```python
from build123d import *

# Parameters (mm, degrees)
CROQUIS2_W                   = 20
CROQUIS2_H                   = 20
SALIENTE_EXTRUIR1_DEPTH      = 50
CROQUIS3_W                   = 20
CROQUIS3_H                   = 20
SALIENTE_EXTRUIR2_DEPTH      = 59
SALIENTE_EXTRUIR4_DEPTH      = 60
SALIENTE_EXTRUIR4_DEPTH_BACK = 20
CROQUIS7_W                   = 30
CROQUIS7_H                   = 10
CROQUIS14_R                  = 12.5
CORTAR_EXTRUIR4_DEPTH        = 5
CROQUIS16_R                  = 2.25
CORTAR_EXTRUIR5_DEPTH        = 10
CROQUIS19_R                  = 1.65
CORTAR_EXTRUIR6_DEPTH        = 10


with BuildPart() as part:
    # Croquis2 → Saliente-Extruir1 (new body)
    with BuildSketch(Plane.XY):
        Rectangle(CROQUIS2_W, CROQUIS2_H)
    extrude(amount=SALIENTE_EXTRUIR1_DEPTH)

    # Croquis3 → Saliente-Extruir2 (add)
    with BuildSketch(Plane(origin=(0, 10, 0), x_dir=(1, 0, 0), z_dir=(0, 1, 0))):
        with Locations((0, -40)):
            Rectangle(CROQUIS3_W, CROQUIS3_H)
    extrude(amount=SALIENTE_EXTRUIR2_DEPTH)

    # Croquis7 → Saliente-Extruir4 (add, two sides: drawn at the far end of the back side and taken through both)
    with BuildSketch(Plane(origin=(0, 0, 30), x_dir=(-1, 0, 0), z_dir=(0, 0, -1)).offset(-SALIENTE_EXTRUIR4_DEPTH_BACK)):
        with Locations((0, 64)):
            Rectangle(CROQUIS7_W, CROQUIS7_H)
    extrude(amount=SALIENTE_EXTRUIR4_DEPTH + SALIENTE_EXTRUIR4_DEPTH_BACK)

    # Croquis14 → Cortar-Extruir4 (cut)
    with BuildSketch(Plane(origin=(0, 69, 0), x_dir=(1, 0, 0), z_dir=(0, 1, 0))):
        with Locations(Location((0, 0, 0), (0, 0, 270))):
            Circle(CROQUIS14_R)
    extrude(amount=-CORTAR_EXTRUIR4_DEPTH, mode=Mode.SUBTRACT)

    # Croquis16 → Cortar-Extruir5 (cut)
    with BuildSketch(Plane(origin=(0, 64, 0), x_dir=(1, 0, 0), z_dir=(0, 1, 0))):
        with Locations(Location((0, 0, 0), (0, 0, 270))):
            Circle(CROQUIS16_R)
    extrude(amount=-CORTAR_EXTRUIR5_DEPTH, mode=Mode.SUBTRACT)

    # Croquis19 → Cortar-Extruir6 (cut)
    with BuildSketch(Plane(origin=(0, 64, 0), x_dir=(1, 0, 0), z_dir=(0, 1, 0))):
        with Locations(Location((8.5, 0, 0), (0, 0, 270))):
            Circle(CROQUIS19_R)
        with Locations(Location((-8.5, 0, 0), (0, 0, 90))):
            Circle(CROQUIS19_R)
    extrude(amount=-CORTAR_EXTRUIR6_DEPTH, mode=Mode.SUBTRACT)


solid = part.part
```
Geometry check sheet. Reference: the model listing, model coordinates, mm. A direction names the side the tool comes from. Coordinates: 2 decimals unless noted, no trailing zeros. Order: outer loops, then holes, each group sorted by start corner. A loop starts at its lowest first (then second) coordinate and runs counter-clockwise, first axis right, second up. Notation, with made-up numbers: (56.5, -0.5) - (77.5, -0.5) arc R8 cw to (77.5, 13.5) - close; hole circle Ø10 at (66.5, -31.75). An arc over 180 degrees is marked (long way). Answer as a JSON object with one key per item and string values. Group by question number.
Item 1: Sectioned sample at C-C, the plane y = -2. Record the cut outline in (x, z), and give its area (3 significant figures).
Item 2: Sectioned sample at B-B, the plane x = 8.5. Record the cut outline in (y, z).
Item 3: Tool access check on faces 1 (the face through (-10, 16, 31)), 2 (the face through (0, 0, 0)), 3 (the face through (3.755, 66.535, 11.923)), 4 (the face through (0, 10, 15)), 5 (the face through (10, 16, 31)). Record the directions out of +Z, -Z, +X, -X, +Y, -Y that give a thin tool (end or side, any length) a straight path to the whole face; none if there is none.
Item 4: Depth check by flat-ended pin: pin 1 Ø2 at (x, y) = (-5, 22.5) entering from -Z; pin 2 Ø10 at (x, y) = (-3.5, 3.5) entering from -Z; pin 3 Ø2 at (x, z) = (8.5, 0) entering from +Y; pin 4 Ø4 at (x, y) = (6, 58) entering from -Z. Enter the tip coordinate at first touch or a pass-through.
Item 5: Sectioned sample at D-D, the plane z = 38. Record the cut outline in (x, y), and give its area (3 significant figures).
Item 6: Sectioned sample at A-A, the plane z = 18. Record the cut outline in (x, y), and give its area (3 significant figures).
Item 7: Draft check along Y on faces 6 (the face through (4, 59, 2)), 7 (the face through (0, 34, 30)), 8 (the face through (15, 64, 11)), 9 (the face through (0, 64, 3)). Enter one of: +Y half, -Y half, draft (parallel to the pull), parting line (faces both ways), or undercut.
Item 8: Scan lines: probe 1 along X at (y, z) = (62.25, 0); probe 2 along Y at (x, z) = (9, 19); probe 3 along Z at (x, y) = (3.25, -6). Record each from-to range of solid material in increasing order.
Resolved:
{
 "1": {"outline": "(-10, 0) - (10, 0) - (10, 50) - (-10, 50) - close", "area": "1,000 mm^2"},
 "2": {"outline": "(-10, 0) - (10, 0) - (10, 30) - (59, 30) - (59, 1.65) - (64, 1.65) - (64, 9.17) - (69, 9.17) - (69, 50) - (-10, 50) - close; (59, -30) - (69, -30) - (69, -9.17) - (64, -9.17) - (64, -1.65) - (59, -1.65) - close"},
 "3": {"face 1": "+Z, -Z, -X, -Y", "face 2": "-Z, +X, -X, -Y", "face 3": "+Y", "face 4": "-Z, +X, -X", "face 5": "+Z, -Z, +X, -Y"},
 "4": {"pin 1": "z = 30", "pin 2": "z = 0", "pin 3": "y = 10", "pin 4": "z = -30"},
 "5": {"outline": "(-15, 59) - (-10, 59) - (-10, -10) - (10, -10) - (10, 59) - (15, 59) - (15, 69) - (-15, 69) - close", "area": "1,680 mm^2"},
 "6": {"outline": "(-15, 59) - (15, 59) - (15, 69) - (-15, 69) - close; (-10, -10) - (10, -10) - (10, 10) - (-10, 10) - close", "area": "700 mm^2"},
 "7": {"face 6": "undercut", "face 7": "undercut", "face 8": "draft", "face 9": "+Y half"},
 "8": {"probe 1": "-15 to -10.15, -6.85 to -2.25, 2.25 to 6.85, 10.15 to 15", "probe 2": "-10 to 10, 59 to 69", "probe 3": "0 to 50"}
}
